For this review, take the finished solid that the model builds, in its own axes (mm). A direction names the side the tool comes from. Give positions to 0.01 mm unless a question says otherwise; leave off trailing zeros. Order: outer loops, then holes, each group sorted by start corner. A loop starts at its lowest first (then second) coordinate and runs counter-clockwise, first axis right, second up.
Item 1: For probe 1 along Y at (x, z) = (0, 5.5); probe 2 along Z at (x, y) = (-7.25, -2); probe 3 along X at (y, z) = (9.5, 1), list the stretches that pass through material, from the lowest coordinate up.
Item 2: Consider section C-C (x = 7.25). Give the boundary of the cut face in (y, z).
Item 3: For P1, Ø1.5, axis at y = 10, z = 2, coming from the +X side; P2, Ø0.8, axis at x = -2.5, z = 6, coming from the -Y side; P3, Ø5, axis at x = 3, z = 2, coming from the -Y side, all flat-tipped, find the tip position at first contact; note any pin that passes through.
Item 4: The part is to be moulded in two halves that separate along Y. For faces 1 (the flat face through (-7, 15.9, -5.5)), 2 (the cylindrical face through (-5.719, -5.594, 0.035)), 3 (the cylindrical face through (-10.2, 13.5, 0.1)), 4 (the cylindrical face through (3.233, -1.341, -4.472)), say which applies: released by +Y, released by -Y, zero draft, split by the parting line, or undercut.
Item 5: Consider section B-B (y = 11.5). Give the boundary of the cut face in (x, z), plus the area to 3 significant figures.
Item 6: Machinability: for faces 5 (the flat face through (0, 10, 4)), 6 (the flat face through (-3, 17, 5.5)), 7 (the flat face through (8, 11, 0)), 8 (the flat face through (0, 0, 6.5)), which of the approach directions +Z, -Z, +X, -X, +Y, -Y give a long, thin tool a straight path to every point of the face, cutting with its end or side? Answer none if there is none.
Autodesk Inventor part; units mm, degrees
ref_plane "YZ Plane" through (0, 0, 0) normal (1, 0, 0) x (0, 1, 0)
ref_plane "XZ Plane" through (0, 0, 0) normal (0, 1, 0) x (-1, 0, 0)
ref_plane "XY Plane" through (0, 0, 0) normal (0, 0, 1) x (1, 0, 0)
sketch "스케치1" plane through (0, 0, 0) normal (0, 0, 1) x (1, 0, 0)
  circle A0 centre (0, 0) radius 3.5
  line L0 (-8, 22) -> (8, 22)
  line L1 (8, 22) -> (8, -8)
  line L2 (8, -8) -> (-8, -8)
  line L3 (-8, -8) -> (-8, 22)
  line L4 (-8, 10) -> (8, 10)
  dimension "d0" = 7
  dimension "d2" = 16
  dimension "d3" = 8
  dimension "d4" = 30
  dimension "d5" = 22
  dimension "d6" = 12
extrude "돌출1" add sketch "스케치1" along normal mid plane 13 contours A0
extrude "돌출2" add sketch "스케치1" along normal mid plane 5 contours L4 L1 L2 L3
extrude "돌출3" add sketch "스케치1" along normal mid plane 13 contours L0 L1 L4 L3
sketch "스케치2" plane through (8, -8, 2.5) normal (1, 0, 0) x (0, 0, -1)
  line L0 (9, 30) -> (-4, 30)
  line L1 (-4, 18) -> (-4, 30)
  point P0 (2.5, 8)
sketch "스케치3" plane through (0, 0, 0) normal (1, 0, 0) x (0, 1, 0)
  circle A0 centre (16, 0) radius 2.5
  line L0 (22, 6.5) -> (22, -6.5)
  line L1 (22, 6.5) -> (10, 6.5)
  point P0 (0, 0)
  dimension "d16" = 5
  dimension "d17" = 6
  dimension "d18" = 6.5
extrude "돌출4" add sketch "스케치3" along normal mid plane 25
fillet "모깎기1" radius 8 2 edges at (8, -8, 0) (-8, -8, 0)
chamfer "모따기1" distance 2 angle 45 4 edges at (8, 16, 6.5) (8, 16, -6.5) (-8, 16, 6.5) (-8, 16, -6.5)
sketch "스케치4" plane through (0, 0, 6.5) normal (0, 0, 1) x (1, 0, 0)
  line L0 (-5.9498, 20.5659) -> (5.0498, 20.5659) construction
  line L1 (5.0498, 20.5659) -> (5.0498, 12.6328) construction
  line L2 (5.0498, 12.6328) -> (-5.9498, 12.6328) construction
  line L3 (-5.9498, 12.6328) -> (-5.9498, 20.5659) construction
  spline S0 degree 2 poles (-0.517, 14.9451) (-0.517, 14.3681) (-0.8866, 13.3827) (-1.2237, 13.0197) knots 0 0 0 1 2 2 2
  spline S1 degree 2 poles (-1.2237, 13.0197) (-1.5608, 12.6566) (-2.5657, 12.2352) (-3.188, 12.2352) knots 0 0 0 1 2 2 2
  spline S2 degree 2 poles (-3.188, 12.2352) (-3.7585, 12.2352) (-4.8736, 12.4881) (-5.282, 12.689) knots 0 0 0 1 2 2 2
  line L4 (-5.282, 12.689) -> (-5.282, 13.8236)
  line L5 (-5.282, 13.8236) -> (-5.2042, 13.8236)
  spline S3 degree 2 poles (-5.2042, 13.8236) (-5.081, 13.7328) (-4.6208, 13.4994) (-4.342, 13.3957) knots 0 0 0 1 2 2 2
  spline S4 degree 2 poles (-4.342, 13.3957) (-4.0243, 13.2855) (-3.4992, 13.1623) (-3.1686, 13.1623) knots 0 0 0 1 2 2 2
  spline S5 degree 2 poles (-3.1686, 13.1623) (-2.8444, 13.1623) (-2.235, 13.3957) (-2.0146, 13.6485) knots 0 0 0 1 2 2 2
  spline S6 degree 2 poles (-2.0146, 13.6485) (-1.8136, 13.8884) (-1.6062, 14.5237) (-1.6062, 14.9516) knots 0 0 0 1 2 2 2
  spline S7 degree 2 poles (-1.6062, 14.9516) (-1.6062, 15.3795) (-1.8396, 15.9241) (-2.06, 16.1056) knots 0 0 0 1 2 2 2
  spline S8 degree 2 poles (-2.06, 16.1056) (-2.2869, 16.3066) (-2.9611, 16.4751) (-3.3695, 16.4751) knots 0 0 0 1 2 2 2
  spline S9 degree 2 poles (-3.3695, 16.4751) (-3.8104, 16.4751) (-4.6856, 16.339) (-4.9514, 16.2806) knots 0 0 0 1 2 2 2
  line L6 (-4.9514, 16.2806) -> (-4.9514, 20.4038)
  line L7 (-4.9514, 20.4038) -> (-0.5624, 20.4038)
  line L8 (-0.5624, 20.4038) -> (-0.5624, 19.4638)
  line L9 (-0.5624, 19.4638) -> (-3.9206, 19.4638)
  line L10 (-3.9206, 19.4638) -> (-3.9206, 17.3309)
  spline S10 degree 2 poles (-3.9206, 17.3309) (-3.7261, 17.3568) (-3.3501, 17.3762) (-3.1945, 17.3762) knots 0 0 0 1 2 2 2
  spline S11 degree 2 poles (-3.1945, 17.3762) (-2.5786, 17.3762) (-1.7293, 17.1753) (-1.3404, 16.8771) knots 0 0 0 1 2 2 2
  spline S12 degree 2 poles (-1.3404, 16.8771) (-0.9449, 16.5788) (-0.517, 15.6712) (-0.517, 14.9451) knots 0 0 0 1 2 2 2
  spline S13 degree 2 poles (5.6159, 16.4038) (5.6159, 14.2514) (4.3647, 12.2352) (3.0616, 12.2352) knots 0 0 0 1 2 2 2
  spline S14 degree 2 poles (3.0616, 12.2352) (1.739, 12.2352) (0.5008, 14.2903) (0.5008, 16.3973) knots 0 0 0 1 2 2 2
  spline S15 degree 2 poles (0.5008, 16.3973) (0.5008, 18.5626) (1.752, 20.5659) (3.0616, 20.5659) knots 0 0 0 1 2 2 2
  spline S16 degree 2 poles (3.0616, 20.5659) (4.3776, 20.5659) (5.6159, 18.4913) (5.6159, 16.4038) knots 0 0 0 1 2 2 2
  spline S17 degree 2 poles (4.2415, 13.9662) (4.3971, 14.3617) (4.5267, 15.5805) (4.5267, 16.4038) knots 0 0 0 1 2 2 2
  spline S18 degree 2 poles (4.5267, 16.4038) (4.5267, 17.2271) (4.3971, 18.4395) (4.235, 18.8479) knots 0 0 0 1 2 2 2
  spline S19 degree 2 poles (4.235, 18.8479) (4.0729, 19.2563) (3.5089, 19.6777) (3.0616, 19.6777) knots 0 0 0 1 2 2 2
  spline S20 degree 2 poles (3.0616, 19.6777) (2.6143, 19.6777) (2.0373, 19.2563) (1.8687, 18.8349) knots 0 0 0 1 2 2 2
  spline S21 degree 2 poles (1.8687, 18.8349) (1.7066, 18.4265) (1.5899, 17.1818) (1.5899, 16.3973) knots 0 0 0 1 2 2 2
  spline S22 degree 2 poles (1.5899, 16.3973) (1.5899, 15.5545) (1.6937, 14.4265) (1.8622, 13.9856) knots 0 0 0 1 2 2 2
  spline S23 degree 2 poles (1.8622, 13.9856) (2.0178, 13.5707) (2.5948, 13.1234) (3.0616, 13.1234) knots 0 0 0 1 2 2 2
  spline S24 degree 2 poles (3.0616, 13.1234) (3.5024, 13.1234) (4.0794, 13.5448) (4.2415, 13.9662) knots 0 0 0 1 2 2 2
  point P0 (0, 0)
extrude "돌출5" cut sketch "스케치4" against normal blind 1
properties part number "1번부품"
Resolved:
1. probe 1: y = -3.5 to 3.5, 10 to 22
1. probe 2: z = -2.5 to 2.5
1. probe 3: x = -8 to 8
2. outline: (-3.38, -2.5) - (10, -2.5) - (10, -5.25) - (22, -5.25) - (22, 5.25) - (10, 5.25) - (10, 2.5) - (-3.38, 2.5) - close
3. P1: stops at x = 8
3. P2: stops at y = -2.8
3. P3: stops at y = -7.98
4. face 1: zero draft
4. face 2: released by -Y
4. face 3: split by the parting line
4. face 4: undercut
5. outline: (-8, -4.5) - (-6, -6.5) - (6, -6.5) - (8, -4.5) - (8, 4.5) - (6, 6.5) - (-6, 6.5) - (-8, 4.5) - close
5. area: 200 mm2
6. face 5: +Z, +X, -X
6. face 6: +Z
6. face 7: +X
6. face 8: +Z, +X, -X, +Y, -Y
